```python
from build123d import *

# Parameters (mm, degrees)
CROQUIS3_R              = 7.5
CROQUIS3_R_2            = 5.5
SALIENTE_EXTRUIR1_DEPTH = 7.5
CROQUIS4_W              = 14.601596012
CROQUIS4_H              = 2.867230366
CORTAR_EXTRUIR1_DEPTH   = 19.5


with BuildPart() as part:
    # Croquis2 → Revolución1 (revolve)
    with BuildSketch(Plane.XY):
        Polygon((-5.5, 0), (-8, 7.5), (-10, 7.5), (-7.5, 0), align=None)
    revolve(axis=Axis((0, 7.5, 0), (0, -1, 0)))

    # Croquis3 → Saliente-Extruir1 (add)
    with BuildSketch(Plane.XZ):
        Circle(CROQUIS3_R)
        Circle(CROQUIS3_R_2, mode=Mode.SUBTRACT)
    extrude(amount=SALIENTE_EXTRUIR1_DEPTH)

    # Croquis4 → Cortar-Extruir1 (cut)
    with BuildSketch(Plane(origin=(0, 7.5, 0), x_dir=(1, 0, 0), z_dir=(0, 1, 0))):
        with Locations((0, 9.433615183)):
            Rectangle(CROQUIS4_W, CROQUIS4_H)
    extrude(amount=-CORTAR_EXTRUIR1_DEPTH, mode=Mode.SUBTRACT)


solid = part.part
```
Model file for the job. Use its own axes, mm. A direction names the side the tool comes from. Coordinates: 2 decimals unless noted, no trailing zeros. Loops run counter-clockwise (first coordinate to the right, second up) from the corner with the lowest first, then second, coordinate; pieces in that order, holes last. Notation, with made-up numbers: M 89,54 L 147,54 A12 ccw 147,58 Z; hole C 24.5,-15.75 d3. An arc over 180 degrees is marked long. Use CSV: the item, a comma, the result in double quotes. Start each with the question number.
1. Flat gauge pins, fed straight in: pin 1 (8 mm diameter, centred on x = -5.5, y = 0.5, fed in from +Z); pin 2 (5 mm diameter, centred on y = -1.5, z = 6, fed in from -X); pin 3 (1 mm diameter, centred on x = -5.5, y = -5.5, fed in from +Z). Where does each tip first touch, or does it go through?
2. Band-saw the part on A-A, the plane z = 0. List the corners of the cut face in (x, y).
3. Tool access for faces 5 (the flat face through (0.7, 7.5, 8.3)), 6 (the cylindrical face through (-7.493, -3.698, 0.33)): list every direction of +Z, -Z, +X, -X, +Y, -Y with a clear straight run to the whole face (end or side of a thin tool).
4. Two-plate mould, pull along Z, no slides. Class faces 1 (the conical face through (-5.9, 2.1, -1.9)), 2 (the cylindrical face through (-1.19, -3.7, -5.37)), 3 (the conical face through (1.712, 1.198, 7.711)), 4 (the flat face through (0, 5, -8)): pulls with the +Z half, pulls with the -Z half, needs draft (parallel to the pull), parting line crosses it, or undercut.
5. Band-saw the part on B-B, the plane y = 2.5. List the corners of the cut face in (x, z), then the cut area to 3 significant figures.
6. Band-saw the part on C-C, the plane y = 6.75. List the corners of the cut face in (x, z), then the cut area to 3 significant figures.
7. Probe probe 1 along X at (y, z) = (-5.25, 0); probe 2 along X at (y, z) = (-1.25, -4.25). List the from-to ranges inside material, lowest first. Write a range as [from, to].
Entries:
1,pin 1,"stops at z = 8.19"
1,pin 2,"stops at x = -6.63"
1,pin 3,"stops at z = 5.59"
2,outline,"M -10,7.5 L -7.5,0 L -7.5,-7.5 L -5.5,-7.5 L -5.5,0 L -8,7.5 Z; M 5.5,-7.5 L 7.5,-7.5 L 7.5,0 L 10,7.5 L 8,7.5 L 5.5,0 Z"
3,face 5,"+Z, -Z, +X, -X, +Y"
3,face 6,"-Y"
4,face 1,"undercut"
4,face 2,"undercut"
4,face 3,"parting line crosses it"
4,face 4,"pulls with the -Z half"
5,outline,"M -2.33,-8 L 2.33,-8 A8.33 ccw long Z; hole C 0,0 d12.67"
5,area,"91.1 mm2"
6,outline,"M -5.57,-8 L 5.57,-8 A9.75 ccw long Z; hole C 0,0 d15.5"
6,area,"96.7 mm2"
7,probe 1,"x = [-7.5, -5.5], [5.5, 7.5]"
7,probe 2,"x = [-6.18, -3.49], [3.49, 6.18]"
